The model under review builds one solid part; all positions refer to its coordinate system, in mm. A direction names the side the tool comes from. Round coordinates to 2 decimals unless told otherwise and drop trailing zeros. Write each loop counter-clockwise with the first axis right and the second up, starting at its lowest first coordinate (ties: lowest second). Pieces come first, ordered by that corner, then holes. Notation, with made-up numbers: (75, -4) - (82, -4) arc R29 ccw to (82, 26) - close; hole circle Ø11 at (84, -36). An arc over 180 degrees is marked (long way). One line per question, with ' | ' between items. Start each with the question number.
```python
from build123d import *

# Parameters (mm, degrees)
BASE_OUTLINE_SKETCH_R          = 1.7
BASE_OUTLINE_SKETCH_R_2        = 1.75
BASE_OUTLINE_SKETCH_R_3        = 6.1
BASE_OUTLINE_DEPTH             = 4
INTERFACE_PROFILE_2_SKETCH_R   = 1.7
INTERFACE_PROFILE_2_SKETCH_R_2 = 6.1
INTERFACE_PROFILE_2_SKETCH_R_3 = 1.1
INTERFACE_PROFILE_2_DEPTH      = 2.4
INTERFACE_PROFILE_3_SKETCH_R   = 6.1
INTERFACE_PROFILE_3_SKETCH_R_2 = 3.1
INTERFACE_PROFILE_3_SKETCH_R_3 = 1.1
INTERFACE_PROFILE_3_DEPTH      = 0.6
INTERFACE_PROFILE_4_SKETCH_R   = 6.1
INTERFACE_PROFILE_4_SKETCH_R_2 = 3.1
INTERFACE_PROFILE_4_DEPTH      = 1


with BuildPart() as part:
    # Base Outline Sketch → Base Outline (new body)
    with BuildSketch(Plane(origin=(0, -157, 0), x_dir=(1, 0, 0), z_dir=(0, 1, 0))):
        with BuildLine():
            Line((-106.291651246, -7), (-64.77693262, -7))
            ThreePointArc((-64.77693262, -7), (-64.069825839, -7.778174593), (-63.291651246, -8.485281374))
            Line((-63.291651246, -8.485281374), (-63.291651246, -50))
            ThreePointArc((-63.291651246, -50), (-56.291651246, -57), (-49.291651246, -50))
            Line((-49.291651246, -50), (-49.291651246, -8.485281374))
            ThreePointArc((-49.291651246, -8.485281374), (-45.291651246, 0), (-49.291651246, 8.485281374))
            Line((-49.291651246, 8.485281374), (-49.291651246, 50))
            ThreePointArc((-49.291651246, 50), (-56.291651246, 57), (-63.291651246, 50))
            Line((-63.291651246, 50), (-63.291651246, 8.485281374))
            ThreePointArc((-63.291651246, 8.485281374), (-64.069825839, 7.778174593), (-64.77693262, 7))
            Line((-64.77693262, 7), (-106.291651246, 7))
            ThreePointArc((-106.291651246, 7), (-113.291651246, 0), (-106.291651246, -7))
        make_face()
        with Locations(Location((-106.291651246, 0, 0), (0, 0, 270))):
            Circle(BASE_OUTLINE_SKETCH_R, mode=Mode.SUBTRACT)
        with Locations(Location((-56.291651246, 50, 0), (0, 0, 270))):
            Circle(BASE_OUTLINE_SKETCH_R, mode=Mode.SUBTRACT)
        with Locations(Location((-56.291651246, 9, 0), (0, 0, 270))):
            Circle(BASE_OUTLINE_SKETCH_R_2, mode=Mode.SUBTRACT)
        with Locations(Location((-65.291651246, 0, 0), (0, 0, 270))):
            Circle(BASE_OUTLINE_SKETCH_R_2, mode=Mode.SUBTRACT)
        with Locations(Location((-56.291651246, 0, 0), (0, 0, 270))):
            Circle(BASE_OUTLINE_SKETCH_R_3, mode=Mode.SUBTRACT)
        with Locations(Location((-56.291651246, -9, 0), (0, 0, 270))):
            Circle(BASE_OUTLINE_SKETCH_R_2, mode=Mode.SUBTRACT)
        with Locations(Location((-56.291651246, -50, 0), (0, 0, 270))):
            Circle(BASE_OUTLINE_SKETCH_R, mode=Mode.SUBTRACT)
    extrude(amount=BASE_OUTLINE_DEPTH)

    # Interface Profile 2 Sketch → Interface Profile 2 (add)
    with BuildSketch(Plane(origin=(0, -153, 0), x_dir=(1, 0, 0), z_dir=(0, 1, 0))):
        with BuildLine():
            Line((-106.291651246, -7), (-64.77693262, -7))
            ThreePointArc((-64.77693262, -7), (-64.069825839, -7.778174593), (-63.291651246, -8.485281374))
            Line((-63.291651246, -8.485281374), (-63.291651246, -50))
            ThreePointArc((-63.291651246, -50), (-56.291651246, -57), (-49.291651246, -50))
            Line((-49.291651246, -50), (-49.291651246, -8.485281374))
            ThreePointArc((-49.291651246, -8.485281374), (-45.291651246, 0), (-49.291651246, 8.485281374))
            Line((-49.291651246, 8.485281374), (-49.291651246, 50))
            ThreePointArc((-49.291651246, 50), (-56.291651246, 57), (-63.291651246, 50))
            Line((-63.291651246, 50), (-63.291651246, 8.485281374))
            ThreePointArc((-63.291651246, 8.485281374), (-64.069825839, 7.778174593), (-64.77693262, 7))
            Line((-64.77693262, 7), (-106.291651246, 7))
            ThreePointArc((-106.291651246, 7), (-113.291651246, 0), (-106.291651246, -7))
        make_face()
        with Locations(Location((-106.291651246, 0, 0), (0, 0, 270))):
            Circle(INTERFACE_PROFILE_2_SKETCH_R, mode=Mode.SUBTRACT)
        with Locations(Location((-56.291651246, 50, 0), (0, 0, 270))):
            Circle(INTERFACE_PROFILE_2_SKETCH_R, mode=Mode.SUBTRACT)
        with Locations(Location((-56.291651246, 0, 0), (0, 0, 270))):
            Circle(INTERFACE_PROFILE_2_SKETCH_R_2, mode=Mode.SUBTRACT)
        with Locations(Location((-56.291651246, -50, 0), (0, 0, 270))):
            Circle(INTERFACE_PROFILE_2_SKETCH_R, mode=Mode.SUBTRACT)
        with Locations(Location((-56.291651246, 9, 0), (0, 0, 270))):
            Circle(INTERFACE_PROFILE_2_SKETCH_R_3, mode=Mode.SUBTRACT)
        with Locations(Location((-65.291651246, 0, 0), (0, 0, 270))):
            Circle(INTERFACE_PROFILE_2_SKETCH_R_3, mode=Mode.SUBTRACT)
        with Locations(Location((-56.291651246, -9, 0), (0, 0, 270))):
            Circle(INTERFACE_PROFILE_2_SKETCH_R_3, mode=Mode.SUBTRACT)
    extrude(amount=INTERFACE_PROFILE_2_DEPTH)

    # Interface Profile 3 Sketch → Interface Profile 3 (add)
    with BuildSketch(Plane(origin=(0, -150.6, 0), x_dir=(1, 0, 0), z_dir=(0, 1, 0))):
        with BuildLine():
            Line((-106.291651246, -7), (-64.77693262, -7))
            ThreePointArc((-64.77693262, -7), (-64.069825839, -7.778174593), (-63.291651246, -8.485281374))
            Line((-63.291651246, -8.485281374), (-63.291651246, -50))
            ThreePointArc((-63.291651246, -50), (-56.291651246, -57), (-49.291651246, -50))
            Line((-49.291651246, -50), (-49.291651246, -8.485281374))
            ThreePointArc((-49.291651246, -8.485281374), (-45.291651246, 0), (-49.291651246, 8.485281374))
            Line((-49.291651246, 8.485281374), (-49.291651246, 50))
            ThreePointArc((-49.291651246, 50), (-56.291651246, 57), (-63.291651246, 50))
            Line((-63.291651246, 50), (-63.291651246, 8.485281374))
            ThreePointArc((-63.291651246, 8.485281374), (-64.069825839, 7.778174593), (-64.77693262, 7))
            Line((-64.77693262, 7), (-106.291651246, 7))
            ThreePointArc((-106.291651246, 7), (-113.291651246, 0), (-106.291651246, -7))
        make_face()
        with Locations(Location((-56.291651246, 0, 0), (0, 0, 270))):
            Circle(INTERFACE_PROFILE_3_SKETCH_R, mode=Mode.SUBTRACT)
        with Locations(Location((-106.291651246, 0, 0), (0, 0, 270))):
            Circle(INTERFACE_PROFILE_3_SKETCH_R_2, mode=Mode.SUBTRACT)
        with Locations(Location((-56.291651246, 50, 0), (0, 0, 270))):
            Circle(INTERFACE_PROFILE_3_SKETCH_R_2, mode=Mode.SUBTRACT)
        with Locations(Location((-56.291651246, -50, 0), (0, 0, 270))):
            Circle(INTERFACE_PROFILE_3_SKETCH_R_2, mode=Mode.SUBTRACT)
        with Locations(Location((-56.291651246, 9, 0), (0, 0, 270))):
            Circle(INTERFACE_PROFILE_3_SKETCH_R_3, mode=Mode.SUBTRACT)
        with Locations(Location((-65.291651246, 0, 0), (0, 0, 270))):
            Circle(INTERFACE_PROFILE_3_SKETCH_R_3, mode=Mode.SUBTRACT)
        with Locations(Location((-56.291651246, -9, 0), (0, 0, 270))):
            Circle(INTERFACE_PROFILE_3_SKETCH_R_3, mode=Mode.SUBTRACT)
    extrude(amount=INTERFACE_PROFILE_3_DEPTH)

    # Interface Profile 4 Sketch → Interface Profile 4 (add)
    with BuildSketch(Plane(origin=(0, -150, 0), x_dir=(1, 0, 0), z_dir=(0, 1, 0))):
        with BuildLine():
            Line((-106.291651246, -7), (-64.77693262, -7))
            ThreePointArc((-64.77693262, -7), (-64.069825839, -7.778174593), (-63.291651246, -8.485281374))
            Line((-63.291651246, -8.485281374), (-63.291651246, -50))
            ThreePointArc((-63.291651246, -50), (-56.291651246, -57), (-49.291651246, -50))
            Line((-49.291651246, -50), (-49.291651246, -8.485281374))
            ThreePointArc((-49.291651246, -8.485281374), (-45.291651246, 0), (-49.291651246, 8.485281374))
            Line((-49.291651246, 8.485281374), (-49.291651246, 50))
            ThreePointArc((-49.291651246, 50), (-56.291651246, 57), (-63.291651246, 50))
            Line((-63.291651246, 50), (-63.291651246, 8.485281374))
            ThreePointArc((-63.291651246, 8.485281374), (-64.069825839, 7.778174593), (-64.77693262, 7))
            Line((-64.77693262, 7), (-106.291651246, 7))
            ThreePointArc((-106.291651246, 7), (-113.291651246, 0), (-106.291651246, -7))
        make_face()
        with Locations(Location((-56.291651246, 0, 0), (0, 0, 270))):
            Circle(INTERFACE_PROFILE_4_SKETCH_R, mode=Mode.SUBTRACT)
        with Locations(Location((-106.291651246, 0, 0), (0, 0, 270))):
            Circle(INTERFACE_PROFILE_4_SKETCH_R_2, mode=Mode.SUBTRACT)
        with Locations(Location((-56.291651246, 50, 0), (0, 0, 270))):
            Circle(INTERFACE_PROFILE_4_SKETCH_R_2, mode=Mode.SUBTRACT)
        with Locations(Location((-56.291651246, -50, 0), (0, 0, 270))):
            Circle(INTERFACE_PROFILE_4_SKETCH_R_2, mode=Mode.SUBTRACT)
    extrude(amount=INTERFACE_PROFILE_4_DEPTH)


solid = part.part
```
1. Add section A-A, the plane z = 0. Write out the cut boundary in (x, y), then the cut area to 3 significant figures.
2. The part is to be moulded in two halves that separate along X. For faces 1 (the face through (-45.292, -153.056, 0.136)), 2 (the face through (-86, -153, 7)), 3 (the face through (-54.557, -155.028, 8.772)), say which applies: pulls with the +X half, pulls with the -X half, needs draft (parallel to the pull), parting line crosses it, or undercut.
3. Wall thickness on line 1 along Z through (x, y) = (-56.5, -155); line 2 along X through (y, z) = (-149.55, 50); line 3 along X through (y, z) = (-156.5, 9): over which ranges is each line inside the solid? List them lowest first. Write a range as [from, to].
4. Add section B-B, the plane x = -96. Write out the cut boundary in (y, z), then the cut area to 3 significant figures.
5. Machinability: for faces 4 (the face through (-109.32, -149.81, -0.67)), 5 (the face through (-63.292, -153, -30)), 6 (the face through (-55.2, -151.52, 8.86)), which of the approach directions +Z, -Z, +X, -X, +Y, -Y give a long, thin tool a straight path to every point of the face, cutting with its end or side? Answer none if there is none.
6. Add section C-C, the plane z = 42.5. Write out the cut boundary in (x, y).
7. Clearance check with flat-ended pins moving along their axes: P1, Ø2.5, axis at y = -153, z = 27.5, coming from the -X side; P2, Ø2, axis at x = -56.29, z = -9, coming from the -Y side; P3, Ø3, axis at x = -56.29, z = 9, coming from the -Y side; P4, Ø10, axis at x = -56.29, z = 0, coming from the +Y side. State where each tip first meets the part, or that it passes through.
Geometry check:
1) outline: (-113.29, -157) - (-107.99, -157) - (-107.99, -150.6) - (-109.39, -150.6) - (-109.39, -149) - (-113.29, -149) - close; (-104.59, -157) - (-67.04, -157) - (-67.04, -153) - (-66.39, -153) - (-66.39, -150) - (-64.19, -150) - (-64.19, -153) - (-63.54, -153) - (-63.54, -157) - (-62.39, -157) - (-62.39, -149) - (-103.19, -149) - (-103.19, -150.6) - (-104.59, -150.6) - close; (-50.19, -157) - (-45.29, -157) - (-45.29, -149) - (-50.19, -149) - close | area: 394 mm2
2) face 1: pulls with the +X half | face 2: needs draft | face 3: undercut
3) line 1: z = [-57, -51.69], [-48.31, -10.74], [-7.26, -6.1], [6.1, 7.26], [10.74, 48.31], [51.69, 57] | line 2: x = [-63.29, -59.39], [-53.19, -49.29] | line 3: x = [-63.29, -58.04], [-54.54, -49.29]
4) outline: (-157, -7) - (-149, -7) - (-149, 7) - (-157, 7) - close | area: 112 mm2
5) face 4: +Y | face 5: -Z, -X, +Y, -Y | face 6: -Y
6) outline: (-63.29, -157) - (-49.29, -157) - (-49.29, -149) - (-63.29, -149) - close
7) P1: stops at x = -63.29 | P2: stops at y = -150 | P3: stops at y = -153 | P4: passes through
